from build123d import *

# Parameters (mm, degrees)
BOSS_EXTRUDE1_DEPTH = 4
BOSS_EXTRUDE1_DRAFT = 10
CUT_EXTRUDE1_START  = 4
SKETCH1_3_R         = 1.1
CUT_EXTRUDE1_DEPTH  = 4
CUT_EXTRUDE2_START  = 4
SKETCH1_4_R         = 8.4
SKETCH1_4_R_2       = 1.1
CUT_EXTRUDE2_DEPTH  = 3


# Read off the part's stored shape, not the designer's step: Boss-Extrude1
with BuildPart() as part:
    # Boss-Extrude1 outline → Boss-Extrude1 (with draft: the straight prism first)
    with BuildSketch(Plane(origin=(0, 4, 0), x_dir=(1, 0, 0), z_dir=(0, 1, 0))):
        with BuildLine():
            ThreePointArc((-58.761875024, -11.799956956), (-58.761875024, -22.494649034), (-49.5, -27.841995072))
            Line((-49.5, -27.841995072), (-9.9, -27.841995072))
            ThreePointArc((-9.9, -27.841995072), (-4.552653961, -26.409178019), (-0.638124976, -22.494649034))
            Line((-0.638124976, -22.494649034), (9.261875024, -5.347346039))
            ThreePointArc((9.261875024, -5.347346039), (9.261875024, 5.347346039), (0, 10.694692077))
            Line((0, 10.694692077), (-39.6, 10.694692077))
            ThreePointArc((-39.6, 10.694692077), (-44.947346039, 9.261875024), (-48.861875024, 5.347346039))
            Line((-48.861875024, 5.347346039), (-58.761875024, -11.799956956))
        make_face()
    extrude(amount=-BOSS_EXTRUDE1_DEPTH)
    # Boss-Extrude1: the draft: its side faces are tilted about the plane it starts from
    boss_extrude1_sides = [part.faces().sort_by_distance(p)[0] for p in [
        (-53.811875024, 2, 3.226305459),
        (-58.761875024, 2, 22.494649033),
        (-29.7, 2, 27.841995072),
        (-4.552653962, 2, 26.409178019),
        (4.311875024, 2, 13.920997536),
        (9.261875024, 2, -5.347346038),
        (-19.8, 2, -10.694692077),
        (-44.947346038, 2, -9.261875024),
    ]]
    draft(boss_extrude1_sides, Plane(origin=(0, 4, 0), x_dir=(1, 0, 0), z_dir=(0, 1, 0)), BOSS_EXTRUDE1_DRAFT)

    # Sketch1<3> → Cut-Extrude1 (cut)
    with BuildSketch(Plane(origin=(0, 0, 0), x_dir=(1, 0, 0), z_dir=(0, 1, 0)).offset(CUT_EXTRUDE1_START)):
        with Locations(Location((-9.9, -17.147302995, 0), (0, 0, 270))):
            Circle(SKETCH1_3_R)
        with Locations(Location((0, 0, 0), (0, 0, 270))):
            Circle(SKETCH1_3_R)
        with Locations(Location((-29.7, -17.147302995, 0), (0, 0, 270))):
            Circle(SKETCH1_3_R)
        with Locations(Location((-39.6, 0, 0), (0, 0, 270))):
            Circle(SKETCH1_3_R)
        with Locations(Location((-49.5, -17.147302995, 0), (0, 0, 270))):
            Circle(SKETCH1_3_R)
        with Locations(Location((-19.8, 0, 0), (0, 0, 270))):
            Circle(SKETCH1_3_R)
    extrude(amount=-CUT_EXTRUDE1_DEPTH, mode=Mode.SUBTRACT)

    # Sketch1<4> → Cut-Extrude2 (cut)
    # profile 1 of 6: a face of its own
    with BuildSketch(Plane(origin=(0, 0, 0), x_dir=(1, 0, 0), z_dir=(0, 1, 0)).offset(CUT_EXTRUDE2_START)):
        with Locations(Location((-19.8, 0, 0), (0, 0, 270))):
            Circle(SKETCH1_4_R)
        with Locations(Location((-19.8, 0, 0), (0, 0, 270))):
            Circle(SKETCH1_4_R_2, mode=Mode.SUBTRACT)
    # profile 2 of 6: a face of its own
    with BuildSketch(Plane(origin=(0, 0, 0), x_dir=(1, 0, 0), z_dir=(0, 1, 0)).offset(CUT_EXTRUDE2_START)):
        with Locations(Location((-9.9, -17.147302995, 0), (0, 0, 270))):
            Circle(SKETCH1_4_R)
        with Locations(Location((-9.9, -17.147302995, 0), (0, 0, 270))):
            Circle(SKETCH1_4_R_2, mode=Mode.SUBTRACT)
    # profile 3 of 6: a face of its own
    with BuildSketch(Plane(origin=(0, 0, 0), x_dir=(1, 0, 0), z_dir=(0, 1, 0)).offset(CUT_EXTRUDE2_START)):
        with Locations(Location((0, 0, 0), (0, 0, 270))):
            Circle(SKETCH1_4_R)
        with Locations(Location((0, 0, 0), (0, 0, 270))):
            Circle(SKETCH1_4_R_2, mode=Mode.SUBTRACT)
    # profile 4 of 6: a face of its own
    with BuildSketch(Plane(origin=(0, 0, 0), x_dir=(1, 0, 0), z_dir=(0, 1, 0)).offset(CUT_EXTRUDE2_START)):
        with Locations(Location((-29.7, -17.147302995, 0), (0, 0, 270))):
            Circle(SKETCH1_4_R)
        with Locations(Location((-29.7, -17.147302995, 0), (0, 0, 270))):
            Circle(SKETCH1_4_R_2, mode=Mode.SUBTRACT)
    # profile 5 of 6: a face of its own
    with BuildSketch(Plane(origin=(0, 0, 0), x_dir=(1, 0, 0), z_dir=(0, 1, 0)).offset(CUT_EXTRUDE2_START)):
        with Locations(Location((-39.6, 0, 0), (0, 0, 270))):
            Circle(SKETCH1_4_R)
        with Locations(Location((-39.6, 0, 0), (0, 0, 270))):
            Circle(SKETCH1_4_R_2, mode=Mode.SUBTRACT)
    # profile 6 of 6: a face of its own
    with BuildSketch(Plane(origin=(0, 0, 0), x_dir=(1, 0, 0), z_dir=(0, 1, 0)).offset(CUT_EXTRUDE2_START)):
        with Locations(Location((-49.5, -17.147302995, 0), (0, 0, 270))):
            Circle(SKETCH1_4_R)
        with Locations(Location((-49.5, -17.147302995, 0), (0, 0, 270))):
            Circle(SKETCH1_4_R_2, mode=Mode.SUBTRACT)
    extrude(amount=-CUT_EXTRUDE2_DEPTH, mode=Mode.SUBTRACT)


solid = part.part
Part model, mm, in its own coordinate system. A direction names the side the tool comes from. Coordinates: 2 decimals unless noted, no trailing zeros. Order: outer loops, then holes, each group sorted by start corner. A loop starts at its lowest first (then second) coordinate and runs counter-clockwise, first axis right, second up. Notation, with made-up numbers: (22, 5.25) - (28, 5.25) arc R15 ccw to (28, 34.25) - close; hole circle Ø4 at (53.5, 51.5). An arc over 180 degrees is marked (long way). Use CSV: the item, a comma, the result in double quotes.
Item 1: Mould opens along Z. For faces 3 (the face through (-41, 1, 0)), 4 (the face through (-25, 0, 8)), 5 (the face through (-59.074, 2.472, 22.49)) say: +Z half, -Z half, draft (parallel to the pull), parting line (faces both ways), or undercut.
Solved:
face 3,"undercut"
face 4,"draft"
face 5,"parting line"
Item 2: Saw through at C-C on y = 3.05. Give the cut face in (x, z), and give its area (3 significant figures).
Solved:
outline,"(-58.91, 11.72) - (-49.01, -5.43) arc R10.86 ccw to (-39.6, -10.86) - (0, -10.86) arc R10.86 ccw to (9.41, 5.43) - (-0.49, 22.58) arc R10.86 ccw to (-9.9, 28.01) - (-49.5, 28.01) arc R10.86 ccw to start; hole circle Ø16.8 at (-49.5, 17.15); hole circle Ø16.8 at (-39.6, 0); hole circle Ø16.8 at (-29.7, 17.15); hole circle Ø16.8 at (-19.8, 0); hole circle Ø16.8 at (-9.9, 17.15); hole circle Ø16.8 at (0, 0)"
area,"1,010 mm²"
Item 3: Drop flat-ended pins along their axis: P1, Ø1, axis at x = -2, z = -4, coming from the +Y side; P2, Ø2, axis at y = 0.5, z = 23.5, coming from the +X side; P3, Ø2, axis at y = 3, z = 12.5, coming from the -X side. Give the stop position or say it passes through.
Solved:
P1,"stops at y = 1"
P2,"stops at x = 0.11"
P3,"stops at x = -59.79"
Item 4: 3-axis set-ups, long thin cutter, end or side, ignore diameter. For faces 1 (the face through (-10.6, 0.5, 16.3)), 2 (the face through (-51, 1, 17)): which of +Z, -Z, +X, -X, +Y, -Y reach the whole face in a straight line?
Solved:
face 1,"+Y, -Y"
face 2,"+Y"
Item 5: Saw through at B-B on z = 0. Give the cut face in (x, y), and give its area (3 significant figures).
Solved:
outline,"(-52.76, 0) - (-40.7, 0) - (-40.7, 1) - (-48, 1) - (-48, 4) - (-51.95, 4) - close; (-38.5, 0) - (-20.9, 0) - (-20.9, 1) - (-28.2, 1) - (-28.2, 4) - (-31.2, 4) - (-31.2, 1) - (-38.5, 1) - close; (-18.7, 0) - (-1.1, 0) - (-1.1, 1) - (-8.4, 1) - (-8.4, 4) - (-11.4, 4) - (-11.4, 1) - (-18.7, 1) - close; (1.1, 0) - (11.4, 0) - (10.69, 4) - (8.4, 4) - (8.4, 1) - (1.1, 1) - close"
area,"95.8 mm²"
Item 6: Saw through at A-A on x = -19.8. Give the cut face in (y, z).
Solved:
outline,"(0, -11.4) - (4, -10.69) - (4, -8.4) - (1, -8.4) - (1, -1.1) - (0, -1.1) - close; (0, 1.1) - (1, 1.1) - (1, 8.4) - (4, 8.4) - (4, 27.84) - (0, 28.55) - close"
Item 7: Probe probe 1 along X at (y, z) = (0.3, 0); probe 2 along X at (y, z) = (1.2, 9.5); probe 3 along Z at (x, y) = (-16, 3.6). List the from-to ranges inside material, lowest first.
Solved:
probe 1,"x = -52.7 to -40.7, -38.5 to -20.9, -18.7 to -1.1, 1.1 to 11.35"
probe 2,"x = -58 to -52.98, -46.02 to -33.18, -26.22 to -13.38, -6.42 to 7.43"
probe 3,"z = -10.77 to -7.49, 7.49 to 11.37, 22.92 to 27.91"
